from build123d import *

# Parameters (mm, degrees)
ESQUISSE1_R        = 3
BOSS_EXTRU_1_DEPTH = 1
CHANFREIN1_SIZE    = 0.75
ESQUISSE2_R        = 2.25
BOSS_EXTRU_2_DEPTH = 10


with BuildPart() as part:
    # Esquisse1 → Boss.-Extru.1 (new body)
    with BuildSketch(Plane.XY):
        Circle(ESQUISSE1_R)
    extrude(amount=BOSS_EXTRU_1_DEPTH)

    # Chanfrein1
    chanfrein1_edges = [part.edges().sort_by_distance(p)[0] for p in [
        (-3, 0, 1),
    ]]
    chamfer(chanfrein1_edges, length=CHANFREIN1_SIZE)

    # Esquisse2 → Boss.-Extru.2 (add)
    with BuildSketch(Plane.XY.offset(1)):
        Circle(ESQUISSE2_R)
    extrude(amount=BOSS_EXTRU_2_DEPTH)


solid = part.part
Can you work these out from the model? Positions are in its coordinate system, mm. A direction names the side the tool comes from. Give positions to 0.01 mm unless a question says otherwise; leave off trailing zeros. Order: outer loops, then holes, each group sorted by start corner. A loop starts at its lowest first (then second) coordinate and runs counter-clockwise, first axis right, second up. Notation, with made-up numbers: M 34,40.25 L 42,40.25 A26 cw 42,60.25 Z; hole C 27.5,4.5 d2. An arc over 180 degrees is marked long. Use a Markdown table: item, result. Add a question column.
Item 1: If I drill on L1, parallel to Y at x = 0.1, z = 9.25; L2, parallel to X at y = -1.2, z = 8.75; L3, parallel to Z at x = 0.45, y = -2.3, over which ranges is the centre line in solid material (lowest first)? Write a range as [from, to].
Item 2: Suppose I cut it at A-A (x = 0). List the corners of the cut face in (y, z) for me, then the cut area to 3 significant figures.
Item 3: Suppose I cut it at C-C (z = 4.75). List the corners of the cut face in (x, y) for me.
Item 4: Will these pins go through, and if not, where does the flat tip stop? pin 1 (1.5 mm diameter, centred on y = 0.5, z = 2.5, fed in from +X); pin 2 (1 mm diameter, centred on y = -2.5, z = 1.5, fed in from +X); pin 3 (1 mm diameter, centred on y = -2, z = 3, fed in from +X); pin 4 (2 mm diameter, centred on x = -0.5, y = -1.5, fed in from -Z).
Item 5: For faces 1 (the cylindrical face through (-0.29, 2.23, 5.93)), 2 (the flat face through (0, 0, 0)), which set-ups out of +Z, -Z, +X, -X, +Y, -Y let a thin tool reach every point of the face, with its end or its side?
Answer sheet:
| question | item | result |
|---|---|---|
| 1 | L1 | y = [-2.25, 2.25] |
| 1 | L2 | x = [-1.9, 1.9] |
| 1 | L3 | z = [0, 0.91] |
| 2 | outline | M -3,0 L 3,0 L 3,0.25 L 2.25,1 L 2.25,11 L -2.25,11 L -2.25,1 L -3,0.25 Z |
| 2 | area | 50.4 mm² |
| 3 | outline | C 0,0 d4.5 |
| 4 | pin 1 | stops at x = 2.25 |
| 4 | pin 2 | stops at x = 1.03 |
| 4 | pin 3 | stops at x = 1.68 |
| 4 | pin 4 | stops at z = 0 |
| 5 | face 1 | +Z |
| 5 | face 2 | -Z, +X, -X, +Y, -Y |
